```python
from build123d import *

# Parameters (mm, degrees)
MODEL_R                   = 3.175
BOSS_EXTRUDE1_DEPTH       = 8.4836
BOSS_EXTRUDE2_DEPTH       = 3.7084
F_4_CLEARANCE_HOLE3_D     = 2.9464
F_4_CLEARANCE_HOLE4_D     = 2.9464
CUT_EXTRUDE1_DEPTH        = 60.573404892
F_6_CLEARANCE_HOLE1_D     = 3.6576
F_6_CLEARANCE_HOLE1_DEPTH = 14.326172531
F_6_CLEARANCE_HOLE1_TIP   = 1.0988539


with BuildPart() as part:
    # Model → Boss-Extrude1 (new body)
    with BuildSketch(Plane.XY):
        with BuildLine():
            Line((30.032015577, -29.521189504), (30.032015577, -26.729824585))
            Line((30.032015577, -26.729824585), (10.04882977, -15.19252688))
            ThreePointArc((10.04882977, -15.19252688), (8.104547287, -14.069994865), (9.227079302, -12.125712382))
            Line((9.227079302, -12.125712382), (29.151876156, 22.3850481))
            Line((29.151876156, 22.3850481), (25.790540116, 39.397524407))
            ThreePointArc((25.790540116, 39.397524407), (13.922877184, 49.944916766), (0.570865514, 41.353485372))
            Line((0.570865514, 41.353485372), (-0.979565285, 37.104375313))
            Line((-0.979565285, 37.104375313), (1.753621818, 35.526369004))
            Line((1.753621818, 35.526369004), (-1.421378182, 30.02710769))
            Line((-1.421378182, 30.02710769), (-3.189468587, 31.047915161))
            Line((-3.189468587, 31.047915161), (-11.768069595, 7.537404491))
            Line((-11.768069595, 7.537404491), (-8.165923931, 5.457704722))
            Line((-8.165923931, 5.457704722), (-11.34077003, -0.041645446))
            Line((-11.34077003, -0.041645446), (-13.977972897, 1.480944339))
            Line((-13.977972897, 1.480944339), (-24.373743148, -27.00969967))
            Line((-24.373743148, -27.00969967), (-20.022585807, -29.521189504))
            Line((-20.022585807, -29.521189504), (30.032015577, -29.521189504))
        make_face()
        with Locations(Location((12.90743615, 36.852072417, 0), (0, 0, 180))):
            Circle(MODEL_R, mode=Mode.SUBTRACT)
    extrude(amount=BOSS_EXTRUDE1_DEPTH)

    # Sketch2 → Boss-Extrude2 (add)
    with BuildSketch(Plane.XY.offset(8.4836)):
        with BuildLine():
            Line((-20.062967478, -15.195589504), (9.227391231, -15.192610427))
            ThreePointArc((9.227391231, -15.192610427), (9.638115998, -15.246619623), (10.04882977, -15.19252688))
            Line((10.04882977, -15.19252688), (30.032015577, -26.729824585))
            Line((30.032015577, -26.729824585), (30.032015577, -29.521189504))
            Line((30.032015577, -29.521189504), (-20.022585807, -29.521189504))
            Line((-20.022585807, -29.521189504), (-24.373743148, -27.00969967))
            Line((-24.373743148, -27.00969967), (-20.062967478, -15.195589504))
        make_face()
    extrude(amount=BOSS_EXTRUDE2_DEPTH)

    # #4 Clearance Hole3 (through all)
    with Locations(Plane(origin=(-14.068152667, 8.12225173, 0), x_dir=(0, 0, 1), z_dir=(-0.8660254037844389, 0.4999999999999996, 0))):
        with Locations((4.2418, 28.46854897)):
            Hole(F_4_CLEARANCE_HOLE3_D / 2)

    # #4 Clearance Hole4 (through all)
    with Locations(Plane(origin=(-8.487819953, 4.900128422, 0), x_dir=(0, 0, 1), z_dir=(-0.8660393963332388, 0.49997576341134725, 0))):
        with Locations((4.2418, -2.53117675)):
            Hole(F_4_CLEARANCE_HOLE4_D / 2)

    # Sketch12 → Cut-Extrude1 (cut, through all)
    with BuildSketch(Plane(origin=(0, 0, 0), x_dir=(-1, 0, 0), z_dir=(0, 0, -1))):
        with BuildLine():
            Line((-15.046182511, -22.675889504), (-9.966182511, -22.675889504))
            ThreePointArc((-9.966182511, -22.675889504), (-8.378682511, -24.263389504), (-9.966182511, -25.850889504))
            Line((-9.966182511, -25.850889504), (-15.046182511, -25.850889504))
            ThreePointArc((-15.046182511, -25.850889504), (-16.633682511, -24.263389504), (-15.046182511, -22.675889504))
        make_face()
        with BuildLine():
            Line((11.894585807, -22.675889504), (16.974585807, -22.675889504))
            ThreePointArc((16.974585807, -22.675889504), (18.562085807, -24.263389504), (16.974585807, -25.850889504))
            Line((16.974585807, -25.850889504), (11.894585807, -25.850889504))
            ThreePointArc((11.894585807, -25.850889504), (10.307085807, -24.263389504), (11.894585807, -22.675889504))
        make_face()
    extrude(amount=-CUT_EXTRUDE1_DEPTH, mode=Mode.SUBTRACT)

    # #6 Clearance Hole1
    with Locations(Plane(origin=(0, -29.521189504, 0), x_dir=(-1, 0, 0), z_dir=(0, -1, 0))):
        with Locations((14.433829056, -6.27141583), (-12.506939307, -6.27141583)):
            Hole(F_6_CLEARANCE_HOLE1_D / 2, depth=F_6_CLEARANCE_HOLE1_DEPTH)
            with Locations((0, 0, -(F_6_CLEARANCE_HOLE1_DEPTH + F_6_CLEARANCE_HOLE1_TIP / 2))):  # 118° drill point
                Cone(0, F_6_CLEARANCE_HOLE1_D / 2, F_6_CLEARANCE_HOLE1_TIP, mode=Mode.SUBTRACT)


solid = part.part
```
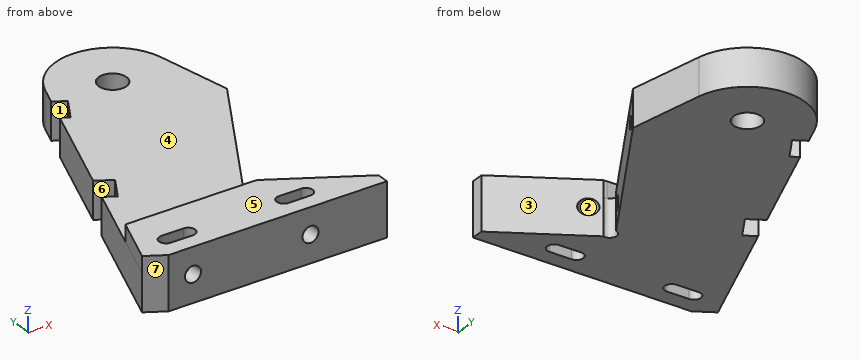
Geometry: final body of the model. Coordinates: model frame, mm. Face numbers are marked on the shaded views. A direction names the side the tool comes from. Coordinates: 2 decimals unless noted, no trailing zeros.
Item 1: Contact query for flat-ended pins moving along their axis: P1, Ø1, axis at x = 5.5, z = 7.5, coming from the +Y side; P2, Ø4, axis at y = -12.5, z = 9, coming from the -X side; P3, Ø1.5, axis at x = -14, z = 4.5, coming from the +Y side. Output: stop coordinate, or through.
Answer:
P1: stops at y = 48.02
P2: stops at x = -19.78
P3: stops at y = 1.48
Item 2: Material intervals for line 1 along Y through (x, z) = (15, 0.75); line 2 along Y through (x, z) = (-15.5, 11.75); line 3 along X through (y, z) = (-23, 8), sorted ascending.
Answer:
line 1: y = -29.52 to -25.85, -22.68 to -18.05, -2.13 to 34.46, 39.24 to 49.82
line 2: y = -29.52 to -25.85, -22.68 to -15.2
line 3: x = -22.91 to -17.94, -10.93 to 9, 16.01 to 23.57
Item 3: Draft query along Y for the marked faces 5, 6 and 7. Return one class per face: released by +Y, released by -Y, zero draft, split by the parting line, or undercut.
Answer:
face 5: zero draft
face 6: undercut
face 7: released by -Y
Item 4: Section query A-A (x = 13.5). State how many separate pieces and enclosed holes the cut face has, then the cut area to 3 significant figures.
Answer:
separate pieces: 6
enclosed holes: 1
area: 487 mm2
Item 5: Access query for the marked faces 1, 2, 3 and 4. Directions: +Z, -Z, +X, -X, +Y, -Y. A direction counts if a zero-diameter tool reaches every point of the face in a straight line with its end or side. Return the directions, or none.
Answer:
face 1: +Z, -Z, -X
face 2: -Y
face 3: +Z, -Z, +X
face 4: +Z, +X, -X, +Y
